Geometry check sheet. Reference: the model listing, model coordinates, mm. Give positions to 0.01 mm unless a question says otherwise; leave off trailing zeros. Write each loop counter-clockwise with the first axis right and the second up, starting at its lowest first coordinate (ties: lowest second). Pieces come first, ordered by that corner, then holes. Notation, with made-up numbers: (65.5, 55.25) -> (111.5, 55.25) arc R35 cw to (111.5, 93.25) -> close; hole circle Ø7 at (62.5, -18.5). An arc over 180 degrees is marked (long way). Write item = value, one per line. Start each with the question number.
1. Cross-section at B-B, the plane z = -44.5. Record the cut outline in (x, y) (3 decimals).
2. Thickness scan on line 1 along X through (y, z) = (-1.5, -27.5) (3 decimals); line 2 along Z through (x, y) = (145.5, -2.2); line 3 along Z through (x, y) = (169, -2.6) (3 decimals). Record the ranges inside material, lowest first.
3. Cross-section at C-C, the plane x = 96. Record the cut outline in (y, z) (3 decimals), plus the area to 3 significant figures.
4. Cross-section at A-A, the plane x = 133.5. Record the cut outline in (y, z) (3 decimals), plus the area to 3 significant figures.
5. Cross-section at D-D, the plane z = -71. Record the cut outline in (x, y) (3 decimals).
6. Depth check by flat-ended pin: P1, Ø1, axis at x = 306, y = -2, coming from the -Z side; P2, Ø1, axis at y = -1.5, z = 1, coming from the -X side; P3, Ø1.6, axis at y = -2, z = -78, coming from the +X side. Enter the tip coordinate at first touch or a pass-through.
```python
from build123d import *

# Parameters (mm, degrees)
F1_DEPTH = 3.175
F2_W     = 88.9
F2_H     = 38.1
F3_DEPTH = 25.4


# Not quite as in the source:
# - a length typed as a fraction of an inch, garbled in the dataset ("3 / 203.2 mm" for 3/8 in), is restored


with BuildPart() as f1:
    # F0 (on Front) → F1 (new body)
    with BuildSketch(Plane.XZ):
        Polygon((50.8, 0), (25.4, 0), (25.4, 3.175), (0, 3.175), (0, 0), (-3.175, 0), (-3.175, -12.7), (0, -12.7), (0, -25.4), (-3.175, -25.4), (-3.175, -38.1), (0, -38.1), (0, -50.8), (-3.175, -50.8), (-3.175, -63.5), (0, -63.5), (0, -76.2), (0, -79.375), (25.4, -79.375), (25.4, -76.2), (50.8, -76.2), (50.8, -79.375), (76.2, -79.375), (76.2, -76.2), (101.6, -76.2), (101.6, -79.375), (127, -79.375), (127, -76.2), (152.4, -76.2), (152.4, -79.375), (177.8, -79.375), (177.8, -76.2), (203.2, -76.2), (203.2, -79.375), (228.6, -79.375), (228.6, -76.2), (254, -76.2), (254, -79.375), (279.4, -79.375), (279.4, -76.2), (304.8, -76.2), (304.8, -63.5), (307.975, -63.5), (307.975, -50.8), (304.8, -50.8), (304.8, -38.1), (307.975, -38.1), (307.975, -25.4), (304.8, -25.4), (304.8, -12.7), (307.975, -12.7), (307.975, 0), (304.8, 0), (279.4, 0), (279.4, 3.175), (254, 3.175), (254, 0), (228.6, 0), (228.6, 3.175), (203.2, 3.175), (203.2, 0), (177.8, 0), (177.8, 3.175), (152.4, 3.175), (152.4, 0), (127, 0), (127, 3.175), (101.6, 3.175), (101.6, 0), (76.2, 0), (76.2, 3.175), (50.8, 3.175), align=None)
    extrude(amount=F1_DEPTH)

    # F2 (on face) → F3 (cut)
    with BuildSketch(Plane.XZ.offset(3.175)):
        with Locations((152.4, -38.1)):
            Rectangle(F2_W, F2_H)
    extrude(amount=-F3_DEPTH, mode=Mode.SUBTRACT)


solid = f1.part
```
Answers:
q1.outline = (0, -3.175) -> (107.95, -3.175) -> (107.95, 0) -> (0, 0) -> close; (196.85, -3.175) -> (304.8, -3.175) -> (304.8, 0) -> (196.85, 0) -> close
q2.line_1 = -3.175 to 107.95, 196.85 to 307.975
q2.line_2 = -76.2 to -57.15, -19.05 to 0
q2.line_3 = -79.375 to -57.15, -19.05 to 3.175
q3.outline = (-3.175, -76.2) -> (0, -76.2) -> (0, 0) -> (-3.175, 0) -> close
q3.area = 242 mm^2
q4.outline = (-3.175, -76.2) -> (0, -76.2) -> (0, -57.15) -> (-3.175, -57.15) -> close; (-3.175, -19.05) -> (0, -19.05) -> (0, 0) -> (-3.175, 0) -> close
q4.area = 121 mm^2
q5.outline = (0, -3.175) -> (304.8, -3.175) -> (304.8, 0) -> (0, 0) -> close
q6.P1 = -63.5
q6.P2 = 0
q6.P3 = 279.4
